```python
from build123d import *

# Parameters (mm, degrees)
SALIENTE_EXTRUIR1_DEPTH = 7
SALIENTE_EXTRUIR2_DEPTH = 7
SALIENTE_EXTRUIR3_DEPTH = 7
REDONDEO1_R             = 10
REDONDEO2_R             = 1
REDONDEO3_R             = 1
CHAFL_N1_SIZE           = 5


with BuildPart() as part:
    # Croquis1 → Saliente-Extruir1 (new body)
    with BuildSketch(Plane.XY.offset(21.250000099)):
        with BuildLine():
            Line((-25.316388353, -1.516889614), (-29.189371699, -1.516889614))
            ThreePointArc((-29.189371699, -1.516889614), (-27.252880026, -9.016889614), (-25.316388353, -1.516889614))
        make_face()
        with BuildLine():
            Line((-26.134846038, -4.016889614), (-28.370914015, -4.016889614))
            ThreePointArc((-28.370914015, -4.016889614), (-27.252880026, -6.516889614), (-26.134846038, -4.016889614))
        make_face(mode=Mode.SUBTRACT)
    extrude(amount=-SALIENTE_EXTRUIR1_DEPTH)

    # Croquis2 → Saliente-Extruir2 (add)
    with BuildSketch(Plane(origin=(0, 0, 14.250000099), x_dir=(-1, 0, 0), z_dir=(0, 0, -1))):
        with BuildLine():
            Line((25.316388353, -1.516889614), (25.316388353, 22.676611236))
            ThreePointArc((25.316388353, 22.676611236), (27.252880026, 22.744234091), (29.189371699, 22.676611236))
            Line((29.189371699, 22.676611236), (29.189371699, -1.516889614))
            Line((29.189371699, -1.516889614), (25.316388353, -1.516889614))
        make_face()
    extrude(amount=-SALIENTE_EXTRUIR2_DEPTH)

    # Croquis3 → Saliente-Extruir3 (add)
    with BuildSketch(Plane(origin=(0, 0, 21.250000099), x_dir=(-1, 0, 0), z_dir=(0, 0, -1))):
        Polygon((25.316388353, 22.676611236), (21.724816583, 21.651922087), (22.905873651, 16.793413653), (25.316388353, 15.869973518), (29.189371699, 15.869973518), (31.599886401, 16.793413653), (32.780943469, 21.651922087), (29.189371699, 22.676611236), align=None)
    extrude(amount=-SALIENTE_EXTRUIR3_DEPTH)

    # Redondeo1
    redondeo1_edges = [part.edges().sort_by_distance(p)[0] for p in [
        (-29.189371699, -1.516889614, 17.750000099),
        (-25.316388353, -1.516889614, 17.750000099),
    ]]
    fillet(redondeo1_edges, radius=REDONDEO1_R)

    # Redondeo2
    redondeo2_edges = [part.edges().sort_by_distance(p)[0] for p in [
        (-25.316388353, 12.487734734, 14.250000099),
        (-29.189371699, 12.487734734, 14.250000099),
        (-27.252880026, -9.016889614, 14.250000099),
        (-29.564906654, -0.415855859, 14.250000099),
        (-24.940853398, -0.415855859, 14.250000099),
    ]]
    fillet(redondeo2_edges, radius=REDONDEO2_R)

    # Redondeo3
    # the kernel refuses this fillet: 1 mm, written as the material it takes off along each edge
    with BuildSketch(Plane(origin=(-25.316388353, 2.298858232, 21.250000099), x_dir=(-1, 0, 0), z_dir=(0, 1, 0)), Plane(origin=(-29.189371699, 15.869973518, 21.250000099), x_dir=(1, 0, 0), z_dir=(0, -1, 0))) as redondeo3_piece_1:
        with BuildLine():
            CenterArc((REDONDEO3_R, -REDONDEO3_R), REDONDEO3_R, 90, 90)
            Line((0, -REDONDEO3_R), (0, 0))
            Line((0, 0), (REDONDEO3_R, 0))
        make_face()
    extrude(amount=13.571115286, mode=Mode.SUBTRACT)
    with BuildSketch(Plane(origin=(-27.252880026, -5.016889614, 21.250000099), x_dir=(-0.8526065480788361, 0.5225534175307739, 0), z_dir=(0.5225534175307739, 0.8526065480788361, 0))) as redondeo3_piece_2:
        with BuildLine():
            CenterArc((4 - REDONDEO3_R, -REDONDEO3_R), REDONDEO3_R, 0, 90)
            Line((4 - REDONDEO3_R, 0), (4, 0))
            Line((4, 0), (4, -REDONDEO3_R))
        make_face()
    revolve(axis=Axis((-27.252880026, -5.016889614, 21.250000099), (0, 0, 1)), revolution_arc=243.007372153, mode=Mode.SUBTRACT)
    with BuildSketch(Plane(origin=(-39.189371699, 2.298858232, 21.250000099), x_dir=(0.8526065480788363, -0.5225534175307737, 0), z_dir=(-0.5225534175307737, -0.8526065480788363, 0))) as redondeo3_piece_3:
        with BuildLine():
            CenterArc((10 + REDONDEO3_R, -REDONDEO3_R), REDONDEO3_R, 90, 90)
            Line((10 + REDONDEO3_R, 0), (10, 0))
            Line((10, 0), (10, -REDONDEO3_R))
        make_face()
    revolve(axis=Axis((-39.189371699, 2.298858232, 21.250000099), (0, 0, 1)), revolution_arc=31.503686076, mode=Mode.SUBTRACT)
    with BuildSketch(Plane(origin=(-15.316388353, 2.298858232, 21.250000099), x_dir=(-0.8526065480788363, -0.5225534175307737, 0), z_dir=(0.5225534175307737, -0.8526065480788363, 0))) as redondeo3_piece_4:
        with BuildLine():
            CenterArc((10 + REDONDEO3_R, REDONDEO3_R), REDONDEO3_R, 180, 90)
            Line((10, REDONDEO3_R), (10, 0))
            Line((10, 0), (10 + REDONDEO3_R, 0))
        make_face()
    revolve(axis=Axis((-15.316388353, 2.298858232, 21.250000099), (0, 0, -1)), revolution_arc=31.503686076, mode=Mode.SUBTRACT)

    # Chaflán1
    # the kernel refuses this chamfer: 5 mm, written as the material it adds along each edge
    with BuildSketch(Plane(origin=(-25.316388353, 3.011558578, 21.250000099), x_dir=(-0.027495876610586317, 0, -0.9996219169112968), z_dir=(0, 1, 0))) as chafl_n1_piece_1_section:
        Polygon((CHAFL_N1_SIZE * 0.999621916911, -CHAFL_N1_SIZE * 0.0274958766106), (-CHAFL_N1_SIZE * 0.0274958766106, -CHAFL_N1_SIZE * 0.999621916911), (0, 0), align=None)
    chafl_n1_piece_1 = extrude(amount=32.523467598, mode=Mode.PRIVATE)
    chafl_n1_piece_1 = chafl_n1_piece_1 & Plane(origin=(-27.252880026, -5.016889614, 17.716506235), x_dir=(0.06975552192119414, 0.997564116817311, 0), z_dir=(0, 0, -1)) * Cylinder(27.761123704, 86, mode=Mode.PRIVATE)
    chafl_n1_piece_1 = split(chafl_n1_piece_1, bisect_by=Plane(origin=(-25.415963135, 15.831827578, 17.716506235), z_dir=(-0.35773655396653403, 0.9338225516425211, 0)), keep=Keep.TOP, mode=Mode.PRIVATE)
    chafl_n1_piece_1 = split(chafl_n1_piece_1, bisect_by=Plane(origin=(-23.262937497, 15.32456193, 17.716506235), z_dir=(-0.9717016867786622, 0.23621141359278705, 0)), keep=Keep.TOP, mode=Mode.PRIVATE)
    chafl_n1_piece_1 = split(chafl_n1_piece_1, bisect_by=Plane(origin=(-23.613600886, 22.190799465, 17.716506235), z_dir=(-0.2743561835557756, -0.9616281425502842, 0)), keep=Keep.TOP, mode=Mode.PRIVATE)
    add(chafl_n1_piece_1)
    with BuildSketch(Plane(origin=(-29.189371699, 35.535026176, 21.250000099), x_dir=(0.027495876610586317, 0, -0.9996219169112968), z_dir=(0, -1, 0))) as chafl_n1_piece_2_section:
        Polygon((CHAFL_N1_SIZE * 0.999621916911, -CHAFL_N1_SIZE * 0.0274958766106), (-CHAFL_N1_SIZE * 0.0274958766106, -CHAFL_N1_SIZE * 0.999621916911), (0, 0), align=None)
    chafl_n1_piece_2 = extrude(amount=32.523467598, mode=Mode.PRIVATE)
    chafl_n1_piece_2 = chafl_n1_piece_2 & Plane(origin=(-27.252880026, -5.016889614, 19.332721103), x_dir=(0.06975552192119414, 0.997564116817311, 0), z_dir=(0, 0, -1)) * Cylinder(27.761123704, 86, mode=Mode.PRIVATE)
    chafl_n1_piece_2 = split(chafl_n1_piece_2, bisect_by=Plane(origin=(-31.36247481, 16.702464034, 19.332721103), z_dir=(0.35773655396653403, 0.9338225516425211, 0)), keep=Keep.TOP, mode=Mode.PRIVATE)
    chafl_n1_piece_2 = split(chafl_n1_piece_2, bisect_by=Plane(origin=(-31.108304124, 22.129132483, 19.332721103), z_dir=(0.2743561835557751, -0.9616281425502844, 0)), keep=Keep.TOP, mode=Mode.PRIVATE)
    chafl_n1_piece_2 = split(chafl_n1_piece_2, bisect_by=Plane(origin=(-32.12707836, 18.962120521, 19.332721103), z_dir=(0.9717016867786619, 0.2362114135927884, 0)), keep=Keep.TOP, mode=Mode.PRIVATE)
    add(chafl_n1_piece_2)


solid = part.part
```
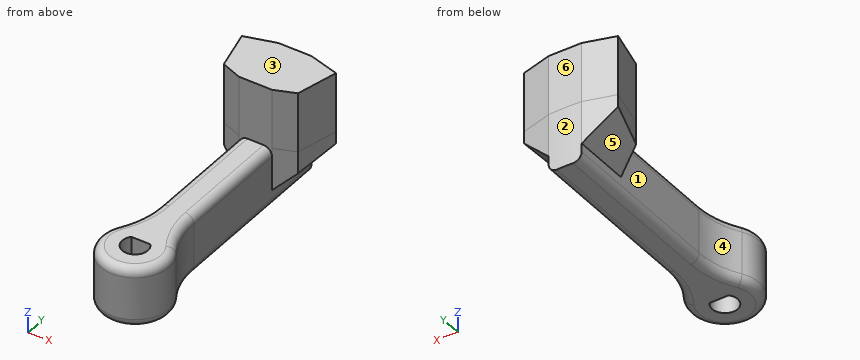
Design review of the part built by this model. Coordinates are the model's own, in mm. Face numbers are marked on the shaded views. A direction names the side the tool comes from. Give positions to 0.01 mm unless a question says otherwise; leave off trailing zeros. Order: outer loops, then holes, each group sorted by start corner. A loop starts at its lowest first (then second) coordinate and runs counter-clockwise, first axis right, second up. Notation, with made-up numbers: (62, -19) -> (105, -19) arc R28 ccw to (105, 20) -> close; hole circle Ø1 at (48, 5.25). An arc over 180 degrees is marked (long way). Write item = value, one per line. Start each with the question number.
(1) We need section A-A on y = 7.5. Write out the cut boundary in (x, z).
(2) Mouldability with a two-part tool opening along Y and no side actions: class the marked faces 1, 2 and 3 as +Y half, -Y half, draft (parallel to the pull), parting line (faces both ways), or undercut.
(3) We need section D-D on y = 19. Write out the cut boundary in (x, z).
(4) We need section B-B on z = 17. Write out the cut boundary in (x, y).
(5) For the marked faces 4, 5 and 6, list the 3-axis set-ups (+Z, -Z, +X, -X, +Y, -Y) from which the entire face can be reached by the end or side of a thin tool; tool diameter is ignored.
(6) We need section C-C on z = 21.75. Write out the cut boundary in (x, y), plus the area to 3 significant figures.
(7) To check wall thickness, follow line 1 along Z through (x, y) = (-26.5, 6); line 2 along Y through (x, z) = (-26.5, 18.75); line 3 along Y through (x, z) = (-29, 27.25). State the ranges of each line that lie inside material, in increasing order.
(8) For pin 1 (4 mm diameter, centred on y = 8, z = 17, fed in from +X); pin 2 (4 mm diameter, centred on x = -27.5, z = 21.5, fed in from +Y); pin 3 (5 mm diameter, centred on y = 2, z = 17, fed in from +X), all flat-tipped, find the tip position at first contact; note any pin that passes through.
Numbers:
q1.outline = (-29.19, 15.25) arc R1 ccw to (-28.19, 14.25) -> (-26.32, 14.25) arc R1 ccw to (-25.32, 15.25) -> (-25.32, 20.25) arc R1 ccw to (-26.32, 21.25) -> (-28.19, 21.25) arc R1 ccw to (-29.19, 20.25) -> close
q2.face_1 = undercut
q2.face_2 = +Y half
q2.face_3 = draft
q3.outline = (-32.14, 19.2) -> (-29.19, 16.25) -> (-29.19, 15.25) arc R1 ccw to (-28.19, 14.25) -> (-26.32, 14.25) arc R1 ccw to (-25.32, 15.25) -> (-25.32, 16.25) -> (-22.37, 19.2) -> (-22.37, 28.25) -> (-32.14, 28.25) -> close
q4.outline = (-30.66, -2.93) arc R4 ccw (long way) to (-23.84, -2.93) arc R10 cw to (-25.32, 2.3) -> (-25.32, 15.87) -> (-24.57, 16.16) -> (-24.57, 22.46) -> (-25.32, 22.68) arc R27.76 ccw to (-29.19, 22.68) -> (-29.94, 22.46) -> (-29.94, 16.16) -> (-29.19, 15.87) -> (-29.19, 2.3) arc R10 cw to start; hole (-28.37, -4.02) arc R1.5 ccw (long way) to (-26.13, -4.02) -> close
q5.face_4 = +Z, -Z, -X
q5.face_5 = -Z, -X, +Y
q5.face_6 = +Z, +X, -X, +Y
q6.outline = (-32.78, 21.65) -> (-31.6, 16.79) -> (-29.19, 15.87) -> (-25.32, 15.87) -> (-22.91, 16.79) -> (-21.72, 21.65) -> (-25.32, 22.68) -> (-29.19, 22.68) -> close
q6.area = 61.4 mm^2
q7.line_1 = 14.25 to 21.25
q7.line_2 = -8.95 to -6.31, -4.02 to 22.73
q7.line_3 = 15.87 to 22.68
q8.pin_1 = -25.32
q8.pin_2 = 22.74
q8.pin_3 = -24.92
